from build123d import *

# Parameters (mm, degrees)
SKETCH1_W           = 38
SKETCH1_H           = 78
SKETCH1_R           = 1.5
SKETCH1_R_2         = 15.5
BOSS_EXTRUDE1_DEPTH = 6.35


with BuildPart() as part:
    # Sketch1 → Boss-Extrude1 (new body)
    with BuildSketch(Plane(origin=(0, 0, 0), x_dir=(1, 0, 0), z_dir=(0, 1, 0))):
        with Locations((19, 39)):
            Rectangle(SKETCH1_W, SKETCH1_H)
        with Locations(Location((4, 4.05, 0), (0, 0, 270))):
            Circle(SKETCH1_R, mode=Mode.SUBTRACT)
        with Locations(Location((34, 4.05, 0), (0, 0, 270))):
            Circle(SKETCH1_R, mode=Mode.SUBTRACT)
        with Locations(Location((34, 34.05, 0), (0, 0, 270))):
            Circle(SKETCH1_R, mode=Mode.SUBTRACT)
        with Locations(Location((4, 34.05, 0), (0, 0, 270))):
            Circle(SKETCH1_R, mode=Mode.SUBTRACT)
        with Locations(Location((19, 19.05, 0), (0, 0, 270))):
            Circle(SKETCH1_R_2, mode=Mode.SUBTRACT)
        with BuildLine():
            Line((4, 72), (4, 52))
            ThreePointArc((4, 52), (6, 50), (8, 52))
            Line((8, 52), (8, 72))
            ThreePointArc((8, 72), (6, 74), (4, 72))
        make_face(mode=Mode.SUBTRACT)
        with BuildLine():
            Line((30, 72), (30, 52))
            ThreePointArc((30, 52), (32, 50), (34, 52))
            Line((34, 52), (34, 72))
            ThreePointArc((34, 72), (32, 74), (30, 72))
        make_face(mode=Mode.SUBTRACT)
    extrude(amount=BOSS_EXTRUDE1_DEPTH)


solid = part.part
Can you work these out from the model? Positions are in its coordinate system, mm. A direction names the side the tool comes from. Coordinates: 2 decimals unless noted, no trailing zeros. Write each loop counter-clockwise with the first axis right and the second up, starting at its lowest first coordinate (ties: lowest second). Pieces come first, ordered by that corner, then holes. Notation, with made-up numbers: (3.5, -17) -> (61.5, -17) arc R24 cw to (61.5, 8) -> close; hole circle Ø11 at (-1, 69). An arc over 180 degrees is marked (long way). Write each question's results on one line, items separated by ' | '. Start each with the question number.
Item 1: If we section it at C-C, the plane y = 1.25: Write out the boundary of the cut face in (x, z), and give its area (3 significant figures).
Item 2: If we section it at A-A, the plane z = -56: Write out the boundary of the cut face in (x, y).
Item 3: Thinking about a two-plate mould opening in Z: for faces 1 (the flat face through (19, 3, 0)), 2 (the flat face through (0, 3, -38)), 3 (the cylindrical face through (34.368, 3.131, -21.068)), which applies, released by +Z, released by -Z, zero draft, split by the parting line, or undercut?
Item 4: If we section it at D-D, the plane z = -19.05: Write out the boundary of the cut face in (x, y).
Item 5: If we section it at B-B, the plane x = 19: Write out the boundary of the cut face in (y, z).
Item 6: On a 3-axis mill with a long thin cutter (end or side, diameter ignored), from which of +Z, -Z, +X, -X, +Y, -Y can I reach the whole of each face in a straight line? I mean faces 4 (the cylindrical face through (32, 3, -74)), 5 (the flat face through (19, 0, -48)). Say none if no direction works.
Item 7: Please list where these lines run through material, in increasing order: probe 1 along X at (y, z) = (3, -62.5); probe 2 along X at (y, z) = (5.25, -19); probe 3 along X at (y, z) = (4.5, -31.5).
Answer block:
1) outline: (0, -78) -> (38, -78) -> (38, 0) -> (0, 0) -> close; hole circle Ø3 at (4, -34.05); hole circle Ø3 at (4, -4.05); hole circle Ø31 at (19, -19.05); hole (4, -72) arc R2 ccw to (8, -72) -> (8, -52) arc R2 ccw to (4, -52) -> close; hole (30, -72) arc R2 ccw to (34, -72) -> (34, -52) arc R2 ccw to (30, -52) -> close; hole circle Ø3 at (34, -34.05); hole circle Ø3 at (34, -4.05) | area: 2,000 mm²
2) outline: (0, 0) -> (4, 0) -> (4, 6.35) -> (0, 6.35) -> close; (8, 0) -> (30, 0) -> (30, 6.35) -> (8, 6.35) -> close; (34, 0) -> (38, 0) -> (38, 6.35) -> (34, 6.35) -> close
3) face 1: released by +Z | face 2: zero draft | face 3: undercut
4) outline: (0, 0) -> (3.5, 0) -> (3.5, 6.35) -> (0, 6.35) -> close; (34.5, 0) -> (38, 0) -> (38, 6.35) -> (34.5, 6.35) -> close
5) outline: (0, -78) -> (6.35, -78) -> (6.35, -34.55) -> (0, -34.55) -> close; (0, -3.55) -> (6.35, -3.55) -> (6.35, 0) -> (0, 0) -> close
6) face 4: +Y, -Y | face 5: +Z, -Z, +X, -X, -Y
7) probe 1: 0 to 4, 8 to 30, 34 to 38 | probe 2: 0 to 3.5, 34.5 to 38 | probe 3: 0 to 9.77, 28.23 to 38
